For this review, take the finished solid that the model builds, in its own axes (mm). Give positions to 0.01 mm unless a question says otherwise; leave off trailing zeros. Order: outer loops, then holes, each group sorted by start corner. A loop starts at its lowest first (then second) coordinate and runs counter-clockwise, first axis right, second up. Notation, with made-up numbers: (-7, 42.5) - (19, 42.5) arc R16 cw to (19, 62.5) - close; hole circle Ø7 at (21.25, -17). An arc over 180 degrees is marked (long way). Answer as a JSON object with one key per item and string values. Group by question number.
from build123d import *

# Parameters (mm, degrees)
SKETCH1_R           = 47.5
SKETCH1_R_2         = 2
SKETCH1_R_3         = 10
SKETCH1_R_4         = 2.1
BOSS_EXTRUDE1_DEPTH = 5


with BuildPart() as part:
    # Sketch1 → Boss-Extrude1 (new body)
    with BuildSketch(Plane(origin=(0, 0, 0), x_dir=(1, 0, 0), z_dir=(0, 1, 0))):
        Circle(SKETCH1_R)
        with Locations((0, 42.5)):
            Circle(SKETCH1_R_2, mode=Mode.SUBTRACT)
        with Locations((40.419901943, 13.133222261)):
            Circle(SKETCH1_R_2, mode=Mode.SUBTRACT)
        with Locations((24.980873222, -34.383222261)):
            Circle(SKETCH1_R_2, mode=Mode.SUBTRACT)
        with Locations((-24.980873222, -34.383222261)):
            Circle(SKETCH1_R_2, mode=Mode.SUBTRACT)
        with Locations((-40.419901943, 13.133222261)):
            Circle(SKETCH1_R_2, mode=Mode.SUBTRACT)
        Circle(SKETCH1_R_3, mode=Mode.SUBTRACT)
        with Locations((-34.595040144, 1.116108173)):
            Circle(SKETCH1_R_4, mode=Mode.SUBTRACT)
        with Locations((14.225114828, -3.421784349)):
            Circle(SKETCH1_R_4, mode=Mode.SUBTRACT)
        with Locations((-33.470320058, -8.820440761)):
            Circle(SKETCH1_R_4, mode=Mode.SUBTRACT)
        with Locations((13.100394742, 6.514764585)):
            Circle(SKETCH1_R_4, mode=Mode.SUBTRACT)
    extrude(amount=BOSS_EXTRUDE1_DEPTH)


solid = part.part
1) Consider section C-C (x = 25.5). Give the boundary of the cut face in (y, z).
2) For line 1 (Z direction, x = 0, y = 2.8); line 2 (X direction, y = 0.85, z = 7.5); line 3 (X direction, y = 3.15, z = 0), list the stretches that pass through material, from the lowest coordinate up.
3) Mouldability with a two-part tool opening along Z and no side actions: class faces 1 (the face through (-10.3, 2.46, 46.37)), 2 (the face through (-24.06, 2.46, 36.16)), 3 (the face through (10, 0, 10)) as released by +Z, released by -Z, zero draft, split by the parting line, or undercut.
4) Consider section B-B (z = -42.5). Give the boundary of the cut face in (x, y).
5) For pin 1 (4 mm diameter, centred on x = 13.1, z = -6.51, fed in from +Y); pin 2 (1.5 mm diameter, centred on x = -15.5, y = 0.5, fed in from +Z); pin 3 (1 mm diameter, centred on y = 4.5, z = 10, fed in from -X), all flat-tipped, find the tip position at first contact; note any pin that passes through.
6) Consider section D-D (y = 4). Give the number of separate pieces and of enclosed holes in the cut face, plus the area to 3 significant figures.
7) Consider section A-A (x = 0). Give the boundary of the cut face in (y, z), plus the area to 3 significant figures.
Result set:
{
 "1": {"outline": "(0, -40.07) - (5, -40.07) - (5, 32.45) - (0, 32.45) - close; (0, 36.31) - (5, 36.31) - (5, 40.07) - (0, 40.07) - close"},
 "2": {"line 1": "z = -47.5 to -44.5, -40.5 to -10, 10 to 47.5", "line 2": "x = -46.9 to -35.1, -31.84 to -6.61, 6.61 to 46.9", "line 3": "x = -47.5 to -36.37, -32.82 to -10, 10 to 47.5"},
 "3": {"face 1": "split by the parting line", "face 2": "undercut", "face 3": "zero draft"},
 "4": {"outline": "(-21.21, 0) - (-2, 0) - (-2, 5) - (-21.21, 5) - close; (2, 0) - (21.21, 0) - (21.21, 5) - (2, 5) - close"},
 "5": {"pin 1": "passes through", "pin 2": "stops at z = 45.15", "pin 3": "stops at x = -46.54"},
 "6": {"separate pieces": "1", "enclosed holes": "10", "area": "6,660 mm2"},
 "7": {"outline": "(0, -47.5) - (5, -47.5) - (5, -44.5) - (0, -44.5) - close; (0, -40.5) - (5, -40.5) - (5, -10) - (0, -10) - close; (0, 10) - (5, 10) - (5, 47.5) - (0, 47.5) - close", "area": "355 mm2"}
}
